from build123d import *

# Parameters (mm, degrees)
F0_R     = 14.5
F0_R_2   = 11.1
F1_DEPTH = 7
F2_R     = 2


with BuildPart() as f1:
    # F0 (on Front) → F1 (new body)
    with BuildSketch(Plane.XZ):
        Polygon((-16.206814, 17.357009), (-23.135017, 29.357009), (-36.991424, 29.357009), (-43.919627, 17.357009), (-36.991424, 5.357009), (-23.135017, 5.357009), align=None)
        Polygon((-34.970698, 25.857009), (-25.155743, 25.857009), (-20.248266, 17.357009), (-25.155743, 8.857009), (-34.970698, 8.857009), (-39.878175, 17.357009), align=None, mode=Mode.SUBTRACT)
        Polygon((-6.928203, 22.714017), (6.928203, 22.714017), (13.856406, 34.714017), (6.928203, 46.714017), (-6.928203, 46.714017), (-13.856406, 34.714017), align=None)
        Polygon((9.814955, 34.714017), (4.907477, 26.214017), (-4.907477, 26.214017), (-9.814955, 34.714017), (-4.907477, 43.214017), (4.907477, 43.214017), align=None, mode=Mode.SUBTRACT)
        Polygon((13.856406, 34.714017), (6.928203, 22.714017), (-6.928203, 22.714017), (-13.856406, 34.714017), (-23.135017, 29.357009), (-16.206814, 17.357009), (-23.135017, 5.357009), (-36.991424, 5.357009), (-36.991424, -5.357009), (-23.135017, -5.357009), (-16.206814, -17.357009), (-23.135017, -29.357009), (-13.856406, -34.714017), (-6.928203, -22.714017), (6.928203, -22.714017), (13.856406, -34.714017), (23.135017, -29.357009), (16.206814, -17.357009), (23.135017, -5.357009), (36.991424, -5.357009), (36.991424, 5.357009), (23.135017, 5.357009), (16.206814, 17.357009), (23.135017, 29.357009), align=None)
        Circle(F0_R, mode=Mode.SUBTRACT)
        Circle(F0_R)
        Circle(F0_R_2, mode=Mode.SUBTRACT)
        Polygon((-23.135017, -5.357009), (-36.991424, -5.357009), (-43.919627, -17.357009), (-36.991424, -29.357009), (-23.135017, -29.357009), (-16.206814, -17.357009), align=None)
        Polygon((-39.878175, -17.357009), (-34.970698, -8.857009), (-25.155743, -8.857009), (-20.248266, -17.357009), (-25.155743, -25.857009), (-34.970698, -25.857009), align=None, mode=Mode.SUBTRACT)
        Polygon((6.928203, -46.714017), (13.856406, -34.714017), (6.928203, -22.714017), (-6.928203, -22.714017), (-13.856406, -34.714017), (-6.928203, -46.714017), align=None)
        Polygon((-4.907477, -43.214017), (-9.814955, -34.714017), (-4.907477, -26.214017), (4.907477, -26.214017), (9.814955, -34.714017), (4.907477, -43.214017), align=None, mode=Mode.SUBTRACT)
        Polygon((43.919627, -17.357009), (36.991424, -5.357009), (23.135017, -5.357009), (16.206814, -17.357009), (23.135017, -29.357009), (36.991424, -29.357009), align=None)
        Polygon((34.970698, -25.857009), (25.155743, -25.857009), (20.248266, -17.357009), (25.155743, -8.857009), (34.970698, -8.857009), (39.878175, -17.357009), align=None, mode=Mode.SUBTRACT)
        Polygon((36.991424, 29.357009), (23.135017, 29.357009), (16.206814, 17.357009), (23.135017, 5.357009), (36.991424, 5.357009), (43.919627, 17.357009), align=None)
        Polygon((39.878175, 17.357009), (34.970698, 8.857009), (25.155743, 8.857009), (20.248266, 17.357009), (25.155743, 25.857009), (34.970698, 25.857009), align=None, mode=Mode.SUBTRACT)
    extrude(amount=F1_DEPTH)

    # F2
    f2_edges = [f1.edges().sort_by_distance(p)[0] for p in [
        (0, -7, 46.714017),
        (10.392305, -7, 40.714017),
        (18.495712, -7, 32.035513),
        (30.063221, -7, 29.357009),
        (40.455525, -7, 23.357009),
        (40.455525, -7, 11.357009),
        (36.991424, -7, 0),
        (40.455525, -7, -11.357009),
        (40.455525, -7, -23.357009),
        (-10.392305, -7, 40.714017),
        (-18.495712, -7, 32.035513),
        (-30.063221, -7, 29.357009),
        (-40.455525, -7, 23.357009),
        (-40.455525, -7, 11.357009),
        (-36.991424, -7, 0),
        (-40.455525, -7, -11.357009),
        (-40.455525, -7, -23.357009),
        (-18.495712, -7, -32.035513),
        (-10.392305, -7, -40.714017),
        (0, -7, -46.714017),
        (10.392305, -7, -40.714017),
        (18.495712, -7, -32.035513),
        (30.063221, -7, -29.357009),
        (-30.063221, -7, -29.357009),
        (0, 0, -46.714017),
        (10.392305, 0, -40.714017),
        (18.495712, 0, -32.035513),
        (30.063221, 0, -29.357009),
        (40.455525, 0, -23.357009),
        (40.455525, 0, -11.357009),
        (36.991424, 0, 0),
        (40.455525, 0, 11.357009),
        (40.455525, 0, 23.357009),
        (30.063221, 0, 29.357009),
        (18.495712, 0, 32.035513),
        (10.392305, 0, 40.714017),
        (0, 0, 46.714017),
        (-10.392305, 0, 40.714017),
        (-18.495712, 0, 32.035513),
        (-30.063221, 0, 29.357009),
        (-40.455525, 0, 23.357009),
        (-40.455525, 0, 11.357009),
        (-36.991424, 0, 0),
        (-40.455525, 0, -11.357009),
        (-40.455525, 0, -23.357009),
        (-30.063221, 0, -29.357009),
        (-18.495712, 0, -32.035513),
        (-10.392305, 0, -40.714017),
    ]]
    fillet(f2_edges, radius=F2_R)


solid = f1.part
Geometry: final body of the model. Coordinates: model frame, mm. A direction names the side the tool comes from. Give positions to 0.01 mm unless a question says otherwise; leave off trailing zeros. Loops run counter-clockwise (first coordinate to the right, second up) from the corner with the lowest first, then second, coordinate; pieces in that order, holes last. Notation, with made-up numbers: (0, 25.25) - (6, 25.25) arc R18 ccw to (6, 55.25) - close; hole circle Ø4 at (11.25, 74). An arc over 180 degrees is marked (long way). One line per question, with ' | ' between items. Start each with the question number.
(1) Section query B-B on x = 0. Return loops of the section in (y, z).
(2) Section query C-C on x = -32. Return loops of the section in (y, z).
(3) Ray query, line 1 (Z direction, x = 0, y = -1.75); line 2 (Z direction, x = 30, y = -3); line 3 (Z direction, x = -2.5, y = -0.5). Return the intervals inside material, ascending. Write a range as from..to.
(4) Section query A-A on z = 0. Return loops of the section in (x, y), then the cut area to 3 significant figures.
(5) Reachability of faces 1 (the flat face through (-22.668, -3.451, 13.167)), 2 (the cylindrical face through (29.695, -0.601, 28.787)), 3 (the flat face through (-30, -3, -29.357)) from +Z, -Z, +X, -X, +Y, -Y: full face, straight path, thin tool, end or side. Return the list, or none.
(6) Contact query for flat-ended pins moving along their axis: pin 1 (3.5 mm diameter, centred on y = -3.5, z = -1, fed in from -X); pin 2 (4 mm diameter, centred on y = -1.5, z = -25, fed in from -X); pin 3 (2 mm diameter, centred on x = -32, y = -4, fed in from +Z). Output: stop coordinate, or through.
(7) Pull-direction query (X, two-part tool) for faces 4 (the flat face through (7.33, -3.45, 39.02)), 5 (the cylindrical face through (39.777, -6.399, -11.323)), 6 (the flat face through (-30, -3, 29.357)); classes: released by +X, released by -X, zero draft, split by the parting line, or undercut.
(8) Section query D-D on z = -24. Count the separate pieces of the cut face and the enclosed holes in it, then the cut area to 3 significant figures.
The answers:
1) outline: (-7, -44.71) arc R2 ccw to (-5, -46.71) - (-2, -46.71) arc R2 ccw to (0, -44.71) - (0, -43.21) - (-7, -43.21) - close; (-7, -26.21) - (0, -26.21) - (0, -11.1) - (-7, -11.1) - close; (-7, 11.1) - (0, 11.1) - (0, 26.21) - (-7, 26.21) - close; (-7, 43.21) - (0, 43.21) - (0, 44.71) arc R2 ccw to (-2, 46.71) - (-5, 46.71) arc R2 ccw to (-7, 44.71) - close
2) outline: (-7, -27.36) arc R2 ccw to (-5, -29.36) - (-2, -29.36) arc R2 ccw to (0, -27.36) - (0, -25.86) - (-7, -25.86) - close; (-7, -8.86) - (0, -8.86) - (0, 8.86) - (-7, 8.86) - close; (-7, 25.86) - (0, 25.86) - (0, 27.36) arc R2 ccw to (-2, 29.36) - (-5, 29.36) arc R2 ccw to (-7, 27.36) - close
3) line 1: -46.7..-43.21, -26.21..-11.1, 11.1..26.21, 43.21..46.7 | line 2: -29.36..-25.86, -8.86..8.86, 25.86..29.36 | line 3: -46.04..-43.21, -26.21..-10.81, 10.81..26.21, 43.21..46.04
4) outline: (-36.99, -5) arc R2 ccw to (-34.99, -7) - (-11.1, -7) - (-11.1, 0) - (-34.99, 0) arc R2 ccw to (-36.99, -2) - close; (11.1, -7) - (34.99, -7) arc R2 ccw to (36.99, -5) - (36.99, -2) arc R2 ccw to (34.99, 0) - (11.1, 0) - close | area: 359 mm2
5) face 1: +Y, -Y | face 2: +Z, +X, +Y | face 3: -Z, -X, +Y, -Y
6) pin 1: x = -36.99 | pin 2: x = -40.64 | pin 3: z = 29.36
7) face 4: undercut | face 5: released by +X | face 6: zero draft
8) separate pieces: 3 | enclosed holes: 0 | area: 390 mm2
